Geometry: final body of the model. Coordinates: model frame, mm. Face numbers are marked on the shaded views. A direction names the side the tool comes from. Coordinates: 2 decimals unless noted, no trailing zeros. Loops run counter-clockwise (first coordinate to the right, second up) from the corner with the lowest first, then second, coordinate; pieces in that order, holes last. Notation, with made-up numbers: (64, 22.5) - (81, 22.5) arc R19 ccw to (81, 28.5) - close; hole circle Ø11 at (-6.75, 77.25). An arc over 180 degrees is marked (long way). Answer in a Markdown table with one row per item.
from build123d import *

# Parameters (mm, degrees)
SKETCH_1_W             = 54
SKETCH_1_H             = 82.2
EXTRUDE_1_DEPTH        = 22
CHAMFER_1_SIZE         = 3.5
SKETCH_2_W             = 54.2
SKETCH_2_H             = 96
EXTRUDE_2_DEPTH        = 12
EXTRUDE_3_DEPTH        = 3.5
CHAMFER_2_SIZE         = 1
SKETCH_5_W             = 9.4
SKETCH_5_H             = 96
SKETCH_5_W_2           = 5.3
SKETCH_5_W_3           = 5.4
SKETCH_5_W_4           = 6.593289258
CUT_EXTRUDE_2_DEPTH    = 9
SKETCH_6_W             = 11
SKETCH_6_H             = 68
CUT_EXTRUDE_3_DEPTH    = 7
SKETCH_7_W             = 8
SKETCH_7_H             = 30
EXTRUDE_5_DEPTH        = 10
SKETCH_8_W             = 15
SKETCH_8_H             = 30.09688029
SKETCH_8_H_2           = 29.900272582
EXTRUDE_6_DEPTH        = 10
SKETCH_9_R             = 1.75
CUT_EXTRUDE_4_DEPTH    = 2
SKETCH_10_W            = 20
SKETCH_10_H            = 2.5
EXTRUDE_7_DEPTH        = 6.8
CUT_EXTRUDE_START      = -5
SKETCH_4_R             = 1.75
CUT_EXTRUDE_1_DEPTH    = 75.485183559
FILLET_1_R             = 2
FILLET_1_OF_MIRROR_1_R = 2


with BuildPart() as part:
    # Эскиз1 → Бобышка-Вытянуть1 (new body)
    with BuildSketch(Plane.XY):
        Rectangle(SKETCH_1_W, SKETCH_1_H)
    extrude(amount=EXTRUDE_1_DEPTH)

    # Фаска1
    chamfer_1_edges = [part.edges().sort_by_distance(p)[0] for p in [
        (0, -41.1, 22),
        (27, 0, 22),
        (0, 41.1, 22),
    ]]
    chamfer(chamfer_1_edges, length=CHAMFER_1_SIZE)

    # Эскиз2 → Бобышка-Вытянуть2 (add)
    with BuildSketch(Plane(origin=(0, 0, 0), x_dir=(-1, 0, 0), z_dir=(0, 0, -1))):
        with Locations((-0.1, 0)):
            Rectangle(SKETCH_2_W, SKETCH_2_H)
    extrude(amount=EXTRUDE_2_DEPTH)

    # Эскиз3 → Бобышка-Вытянуть3 (add)
    with BuildSketch(Plane.ZY.offset(27)):
        with BuildLine():
            Line((-12, 48), (11.75, 48))
            Line((11.75, 48), (11.75, 44))
            ThreePointArc((11.75, 44), (14, 41.75), (16.25, 44))
            Line((16.25, 44), (16.25, 48))
            Line((16.25, 48), (25.5, 48))
            Line((25.5, 48), (25.5, -48))
            Line((25.5, -48), (16.25, -48))
            Line((16.25, -48), (16.25, -44))
            ThreePointArc((16.25, -44), (14, -41.75), (11.75, -44))
            Line((11.75, -44), (11.75, -48))
            Line((11.75, -48), (-12, -48))
            Line((-12, -48), (-12, 48))
        make_face()
    extrude(amount=EXTRUDE_3_DEPTH)

    # Фаска2
    chamfer_2_edges = [part.edges().sort_by_distance(p)[0] for p in [
        (-28.75, -48, 25.5),
        (-28.75, 48, 25.5),
    ]]
    chamfer(chamfer_2_edges, length=CHAMFER_2_SIZE)

    # Эскиз5 → Вырез-Вытянуть2 (cut)
    with BuildSketch(Plane(origin=(0, 0, -12), x_dir=(-1, 0, 0), z_dir=(0, 0, -1))):
        with Locations((22.8, 0)):
            Rectangle(SKETCH_5_W, SKETCH_5_H)
        with Locations((14.65, 0)):
            Rectangle(SKETCH_5_W_2, SKETCH_5_H)
        with Locations((8.5, 0)):
            Rectangle(SKETCH_5_W_3, SKETCH_5_H)
        with Locations((2.3, 0)):
            Rectangle(SKETCH_5_W_3, SKETCH_5_H)
        with Locations((-3.9, 0)):
            Rectangle(SKETCH_5_W_3, SKETCH_5_H)
        with Locations((-10.1, 0)):
            Rectangle(SKETCH_5_W_3, SKETCH_5_H)
        with Locations((-16.3, 0)):
            Rectangle(SKETCH_5_W_3, SKETCH_5_H)
        with Locations((-23.096644629, 0)):
            Rectangle(SKETCH_5_W_4, SKETCH_5_H)
    extrude(amount=-CUT_EXTRUDE_2_DEPTH, mode=Mode.SUBTRACT)

    # Эскиз6 → Вырез-Вытянуть3 (cut)
    with BuildSketch(Plane(origin=(27, 0, 0), x_dir=(0, 0, -1), z_dir=(1, 0, 0))):
        with Locations((-11.5, 0)):
            Rectangle(SKETCH_6_W, SKETCH_6_H)
    extrude(amount=-CUT_EXTRUDE_3_DEPTH, mode=Mode.SUBTRACT)

    # Эскиз7 → Бобышка-Вытянуть5 (add)
    with BuildSketch(Plane(origin=(20, 0, 0), x_dir=(0, 0, -1), z_dir=(1, 0, 0))):
        with Locations((-10.5, -15.05)):
            Rectangle(SKETCH_7_W, SKETCH_7_H)
        with Locations((-10.5, 15.05)):
            Rectangle(SKETCH_7_W, SKETCH_7_H)
    extrude(amount=EXTRUDE_5_DEPTH)

    # Эскиз8 → Бобышка-Вытянуть6 (add)
    with BuildSketch(Plane(origin=(30, 0, 0), x_dir=(0, 0, -1), z_dir=(1, 0, 0))):
        with Locations((-14, -15.001559855)):
            Rectangle(SKETCH_8_W, SKETCH_8_H)
        with Locations((-14, 15.099863709)):
            Rectangle(SKETCH_8_W, SKETCH_8_H_2)
    extrude(amount=EXTRUDE_6_DEPTH)

    # Эскиз9 → Вырез-Вытянуть4 (cut)
    with BuildSketch(Plane(origin=(40, 0, 0), x_dir=(0, 0, -1), z_dir=(1, 0, 0))):
        with Locations((-18.5, -27.55)):
            Circle(SKETCH_9_R)
        with Locations((-18.5, -22.55)):
            Circle(SKETCH_9_R)
        with Locations((-18.5, -17.55)):
            Circle(SKETCH_9_R)
        with Locations((-18.5, -12.55)):
            Circle(SKETCH_9_R)
        with Locations((-18.5, -7.55)):
            Circle(SKETCH_9_R)
        with Locations((-18.5, -2.55)):
            Circle(SKETCH_9_R)
        with Locations((-18.5, 2.55)):
            Circle(SKETCH_9_R)
        with Locations((-18.5, 7.55)):
            Circle(SKETCH_9_R)
        with Locations((-18.5, 12.55)):
            Circle(SKETCH_9_R)
        with Locations((-18.5, 17.55)):
            Circle(SKETCH_9_R)
        with Locations((-18.5, 22.55)):
            Circle(SKETCH_9_R)
        with Locations((-18.5, 27.55)):
            Circle(SKETCH_9_R)
    extrude(amount=-CUT_EXTRUDE_4_DEPTH, mode=Mode.SUBTRACT)

    # Эскиз10 → Бобышка-Вытянуть7 (add)
    with BuildSketch(Plane(origin=(0, 41.1, 0), x_dir=(1, 0, 0), z_dir=(0, 1, 0))):
        with Locations((0, -1.25)):
            Rectangle(SKETCH_10_W, SKETCH_10_H)
    extrude_7 = extrude(amount=EXTRUDE_7_DEPTH)

    # Эскиз4 → Вырез-Вытянуть1 (cut)
    with BuildSketch(Plane.XY.offset(CUT_EXTRUDE_START)):
        with Locations(Location((0.7, -44, 0), (0, 0, 99.870889606))):
            Circle(SKETCH_4_R)
        with Locations(Location((0.7, 44, 0), (0, 0, 180))):
            Circle(SKETCH_4_R)
    cut_extrude_1 = extrude(amount=CUT_EXTRUDE_1_DEPTH, mode=Mode.SUBTRACT)

    # Скругление1
    fillet_1_edges = [part.edges().sort_by_distance(p)[0] for p in [
        (10, 47.9, 1.25),
        (-10, 47.9, 1.25),
    ]]
    fillet(fillet_1_edges, radius=FILLET_1_R)

    # Зеркальное отражение1: Бобышка-Вытянуть7, Вырез-Вытянуть1 across plane
    add(extrude_7.mirror(Plane.ZX))
    add(cut_extrude_1.mirror(Plane.ZX), mode=Mode.SUBTRACT)

    # Скругление1 of Зеркальное отражение1
    fillet_1_of_mirror_1_edges = [part.edges().sort_by_distance(p)[0] for p in [
        (10, -47.9, 1.25),
        (-10, -47.9, 1.25),
    ]]
    fillet(fillet_1_of_mirror_1_edges, radius=FILLET_1_OF_MIRROR_1_R)


solid = part.part
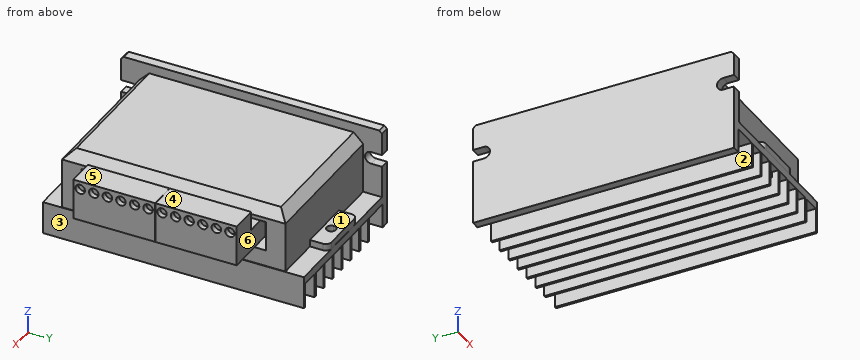
(1) Cut plane A-A on x = 21. Output: boundary loops of the cut face in (y, z), then the cut area to 3 significant figures.
Verdict:
| item | result |
|---|---|
| outline | (-48, -3) - (48, -3) - (48, 0) - (41.1, 0) - (41.1, 18.5) - (37.6, 22) - (-37.6, 22) - (-41.1, 18.5) - (-41.1, 0) - (-48, 0) - close; (-30.05, 6.5) - (-0.05, 6.5) - (-0.05, 14.5) - (-30.05, 14.5) - close; (0.05, 6.5) - (30.05, 6.5) - (30.05, 14.5) - (0.05, 14.5) - close; hole (-34, 6) - (34, 6) - (34, 17) - (-34, 17) - close |
| area | 1,820 mm² |
(2) First-contact query: pin 1 Ø1.8 at (y, z) = (-12.5, 19) entering from +X; pin 2 Ø2.5 at (x, y) = (-7.5, 10) entering from -Z; pin 3 Ø4 at (x, y) = (0.7, -44) entering from +Z. Flat tips, straight axial feed; report the tip coordinate or a pass-through.
Verdict:
| item | result |
|---|---|
| pin 1 | stops at x = 38 |
| pin 2 | stops at z = -3 |
| pin 3 | stops at z = 2.5 |
(3) Cut plane C-C on x = 4. Output: boundary loops of the cut face in (y, z), then the cut area to 3 significant figures.
Verdict:
| item | result |
|---|---|
| outline | (-48, -3) - (48, -3) - (48, 0) - (47.9, 0) - (47.9, 2.5) - (41.1, 2.5) - (41.1, 18.5) - (37.6, 22) - (-37.6, 22) - (-41.1, 18.5) - (-41.1, 2.5) - (-47.9, 2.5) - (-47.9, 0) - (-48, 0) - close |
| area | 2,120 mm² |
(4) Access query for the marked faces 1, 2, 3 and 4. Directions: +Z, -Z, +X, -X, +Y, -Y. A direction counts if a zero-diameter tool reaches every point of the face in a straight line with its end or side. Return the directions, or none.
Verdict:
| item | result |
|---|---|
| face 1 | +Z, +X, +Y |
| face 2 | -Z, +Y, -Y |
| face 3 | -Z, +X, +Y, -Y |
| face 4 | +Z, +X, +Y, -Y |
(5) Cut plane D-D on z = -7. State how many separate pieces and enclosed holes the cut face has, then the cut area to 3 significant figures.
Verdict:
| item | result |
|---|---|
| separate pieces | 9 |
| enclosed holes | 0 |
| area | 903 mm² |
(6) Cut plane B-B on x = 35.5. Output: boundary loops of the cut face in (y, z).
Verdict:
| item | result |
|---|---|
| outline | (-30.05, 6.5) - (0.05, 6.5) - (0.05, 21.5) - (-30.05, 21.5) - close; (0.15, 6.5) - (30.05, 6.5) - (30.05, 21.5) - (0.15, 21.5) - close |
(7) Ray query, probe 1 along X at (y, z) = (-44, 1); probe 2 along Y at (x, z) = (0.7, 1.75); probe 3 along X at (y, z) = (-44, -2). Return the intervals inside material, ascending.
Verdict:
| item | result |
|---|---|
| probe 1 | x = -30.5 to -27, -10 to -1.05, 2.45 to 10 |
| probe 2 | y = -47.9 to -45.75, -42.25 to 42.25, 45.75 to 47.9 |
| probe 3 | x = -30.5 to -1.05, 2.45 to 27.2 |
(8) Pull-direction query (Y, two-part tool) for the marked faces 5 and 6; classes: pulls with the +Y half, pulls with the -Y half, needs draft (parallel to the pull), parting line crosses it, or undercut.
Verdict:
| item | result |
|---|---|
| face 5 | needs draft |
| face 6 | undercut |
